Could you check a few things on this model? Use its own coordinates, in mm. A direction names the side the tool comes from. Give positions to 0.01 mm unless a question says otherwise; leave off trailing zeros. Loops run counter-clockwise (first coordinate to the right, second up) from the corner with the lowest first, then second, coordinate; pieces in that order, holes last. Notation, with made-up numbers: M 46,21 L 57,21 A31 cw 57,49 Z; hole C -32,50.25 d6. An arc over 180 degrees is marked long. Write each question's results on one line, items separated by ' | '. Start each with the question number.
from build123d import *

# Parameters (mm, degrees)
F0_W     = 203.2
F0_H     = 304.8
F1_DEPTH = 12.7
F2_W     = 241.3
F2_H     = 342.9
F3_DEPTH = 19.05
F4_W     = 241.3
F4_H     = 19.05
F5_DEPTH = 19.05
F6_R     = 3.175
F7_DEPTH = 25.4


with BuildPart() as f1:
    # F0 (on Top) → F1 (new body)
    with BuildSketch(Plane.XY):
        Rectangle(F0_W, F0_H)
    extrude(amount=F1_DEPTH)

    # F2 (on face) → F3 (join)
    with BuildSketch(Plane(origin=(0, 0, 0), x_dir=(1, 0, 0), z_dir=(0, 0, -1))):
        with Locations((0, -19.05)):
            Rectangle(F2_W, F2_H)
    extrude(amount=F3_DEPTH)

    # F4 (on face) → F5 (join)
    with BuildSketch(Plane(origin=(0, 0, -19.05), x_dir=(1, 0, 0), z_dir=(0, 0, -1))):
        with Locations((0, -180.975)):
            Rectangle(F4_W, F4_H)
    extrude(amount=F5_DEPTH)

    # F6 (on face) → F7 (cut)
    with BuildSketch(Plane.XY):
        with Locations((0, 161.925)):
            Circle(F6_R)
        with Locations((111.125, 101.6)):
            Circle(F6_R)
        with Locations((111.125, -101.6)):
            Circle(F6_R)
        with Locations((111.125, 0)):
            Circle(F6_R)
        with Locations((-111.125, 101.6)):
            Circle(F6_R)
        with Locations((-111.125, 0)):
            Circle(F6_R)
        with Locations((-111.125, -101.6)):
            Circle(F6_R)
    extrude(amount=-F7_DEPTH, mode=Mode.SUBTRACT)


solid = f1.part
1) If we section it at A-A on x = -45: Write out the boundary of the cut face in (y, z), plus the area to 3 significant figures.
2) If we section it at B-B on y = -38.5: Write out the boundary of the cut face in (x, z).
3) If we section it at D-D on z = -29: Write out the boundary of the cut face in (x, y).
4) Thinking about a two-plate mould opening in X: for faces 6 (the face through (-120.65, 21, -10)), 7 (the face through (-1, 2, 12.7)), 8 (the face through (-108.097, 0.954, -9.392)), 9 (the face through (-0.413, 165.073, -9.392)), which applies, pulls with the +X half, pulls with the -X half, needs draft (parallel to the pull), parting line crosses it, or undercut?
5) Please list where these lines run through material, in increasing order: line 1 (X direction, y = -101, z = -4); line 2 (Z direction, x = 11, y = 12); line 3 (X direction, y = 87, z = 7). Write a range as from..to.
6) I'm going to push flat-ended pins straight in: P1, Ø1.5, axis at x = 58, y = 73, coming from the -Z side; P2, Ø10, axis at x = -17.5, z = -22, coming from the -Y side; P3, Ø6.5, axis at x = 50.5, z = 8.5, coming from the +Y side; P4, Ø5, axis at x = 111.125, y = -101.6, coming from the +Z side. Where does each tip first touch, or does it pass through?
7) Which directions (+Z, -Z, +X, -X, +Y, -Y) give clear straight access to the entire face, cutting with the end or side of a thin tool? Please do faces 1 (the face through (-1, 152.4, 6)), 2 (the face through (101.6, -2, 6)), 3 (the face through (-101.6, -2, 6)), 4 (the face through (114.153, 102.554, -9.392)), 5 (the face through (-2, 7, -19.05)).
8) If we section it at C-C on z = 7.5: Write out the boundary of the cut face in (x, y), plus the area to 3 significant figures.
Calculated:
1) outline: M -152.4,-19.05 L 171.45,-19.05 L 171.45,-38.1 L 190.5,-38.1 L 190.5,0 L 152.4,0 L 152.4,12.7 L -152.4,12.7 Z | area: 10,800 mm2
2) outline: M -120.65,-19.05 L 120.65,-19.05 L 120.65,0 L 101.6,0 L 101.6,12.7 L -101.6,12.7 L -101.6,0 L -120.65,0 Z
3) outline: M -120.65,171.45 L 120.65,171.45 L 120.65,190.5 L -120.65,190.5 Z
4) face 6: pulls with the -X half | face 7: needs draft | face 8: undercut | face 9: undercut
5) line 1: x = -120.65..-114.24, -108.01..108.01, 114.24..120.65 | line 2: z = -19.05..12.7 | line 3: x = -101.6..101.6
6) P1: stops at z = -19.05 | P2: stops at y = -152.4 | P3: stops at y = 152.4 | P4: passes through
7) face 1: +Z, +X, -X, +Y | face 2: +Z, +X, +Y, -Y | face 3: +Z, -X, +Y, -Y | face 4: +Z, -Z | face 5: -Z, +X, -X, -Y
8) outline: M -101.6,-152.4 L 101.6,-152.4 L 101.6,152.4 L -101.6,152.4 Z | area: 61,900 mm2
